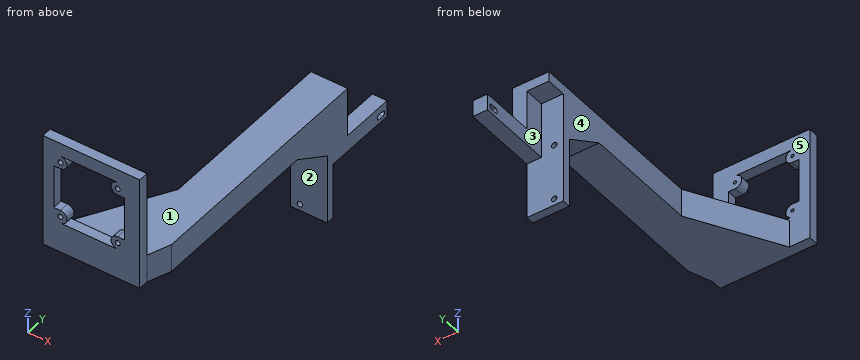
Autodesk Inventor part; units mm, degrees
ref_plane "YZ Plane" through (0, 0, 0) normal (1, 0, 0) x (0, 1, 0)
ref_plane "XZ Plane" through (0, 0, 0) normal (0, 1, 0) x (-1, 0, 0)
ref_plane "XY Plane" through (0, 0, 0) normal (0, 0, 1) x (1, 0, 0)
sketch "Sketch1" plane through (0, 0, 0) normal (0, 1, 0) x (-1, 0, 0)
  line L0 (0, 0) -> (13, 0)
  line L1 (13, 0) -> (13, -44)
  line L2 (13, -44) -> (0, -44)
  line L3 (0, -44) -> (0, 0)
  line L4 (13, 0) -> (13, -6)
  line L5 (13, -6) -> (7.5, -6)
  line L6 (7.5, -6) -> (7.5, -40)
  circle A0 centre (7.5, -6) radius 1.65
  circle A1 centre (7.5, -40) radius 1.65
  dimension "d0" = 13
  dimension "d1" = 44
  dimension "d2" = 6
  dimension "d3" = 5.5
  dimension "d4" = 34
  dimension "d5" = 3.3
  dimension "d6" = 3.3
extrude "Extrusion1" add sketch "Sketch1" along normal blind 5
sketch "Sketch2" plane through (0, 0, 0) normal (1, 0, 0) x (0, 0, -1)
  line L0 (0, 5) -> (44, 5)
  line L1 (0, 5) -> (44, 5)
  line L2 (44, 5) -> (44, 50)
  line L3 (44, 50) -> (0, 50)
  line L4 (0, 50) -> (0, 5)
  line L5 (0, 0) -> (44, 0)
  line L6 (44, 0) -> (44, 5)
  line L7 (44, 5) -> (0, 5)
  line L8 (0, 5) -> (0, 0)
  line L9 (0, 50) -> (10, 50)
  line L10 (10, 50) -> (10, 5)
  line L11 (10, 5) -> (0, 5)
  line L12 (0, 5) -> (0, 50)
  dimension "d9" = 44
  dimension "d10" = 45
  dimension "d11" = 10
extrude "Extrusion2" add sketch "Sketch2" along normal blind 4 contours L4 L3 L10 L0 | L0 L6 L5 L8
sketch "Sketch3" plane through (4, 0, 0) normal (1, 0, 0) x (0, 0, -1)
  line L0 (44, 5) -> (10, 5)
  line L1 (10, 5) -> (10, 45)
  line L2 (10, 5) -> (10, 50)
  line L3 (0, 50) -> (0, 5)
  line L4 (0, 45) -> (4.4, 45)
  line L5 (6, 45) -> (6, 46.5)
  line L6 (6, 45) -> (6, 43.5)
  line L7 (4.4, 46.5) -> (4.4, 43.5)
  line L8 (7.6, 46.5) -> (7.6, 43.5)
  arc A0 (5.4432, 45) -> (6, 44.9) centre (6, 46.5) ccw
  arc A1 (6.5568, 45) -> (4.4, 46.5) centre (6, 46.5) ccw
  line L9 (10, 45) -> (6.5568, 45)
  line L10 (5.4432, 45) -> (0, 45)
  arc A2 (6, 45.1) -> (5.4432, 45) centre (6, 43.5) ccw
  arc A3 (4.4, 43.5) -> (7.6, 43.5) centre (6, 43.5) ccw
  point P0 (0, 0)
  dimension "d14" = 40
  dimension "d15" = 6
  dimension "d16" = 1.5
  dimension "d17" = 1.5
extrude "Extrusion3" cut sketch "Sketch3" against normal blind 4 contours L6 A0 A2 L5 | A1 L9 L8 A3 L7 | L8 L9 A1
sketch "Sketch4" plane through (-13, 0, 0) normal (0, 0, 1) x (1, 0, 0)
  line L0 (0, 0) -> (17, 0)
  line L1 (17, 0) -> (17, 5)
  line L2 (0, 0) -> (17, 0)
  line L3 (17, 0) -> (17, 5)
  line L4 (17, 5) -> (0, 5)
  line L5 (0, 5) -> (0, 0)
  line L6 (13, 50) -> (13, 5)
  line L7 (17, 0) -> (13, 0)
  line L8 (13, 0) -> (13, 17)
  line L9 (13, 17) -> (17, 17)
  line L10 (17, 17) -> (17, 0)
  dimension "d22" = 17
extrude "Extrusion4" add sketch "Sketch4" along normal blind 30
sketch "Sketch5" plane through (0, 0, 0) normal (0, -1, 0) x (1, 0, 0)
  line L0 (-13, -44) -> (-13, 30)
  line L1 (-13, 30) -> (4, 30)
  line L2 (4, 30) -> (4, 13)
  line L3 (4, 13) -> (-13, 13)
  line L4 (-13, 13) -> (-13, 30)
  point P0 (0, 0)
  dimension "d25" = 17
  dimension "d26" = 17
extrude "Extrusion5" add sketch "Sketch5" along normal blind 150
sketch "Sketch7" plane through (0, -150, 0) normal (0, -1, 0) x (1, 0, 0)
  line L0 (4, 13) -> (-13, 13)
  line L1 (0, 30) -> (0, -10)
  line L2 (0, 13) -> (0, 30)
  line L3 (0, 30) -> (0, 52.6)
  circle A0 centre (-36, 52.6) radius 9
  line L4 (-36, 52.6) -> (-36, 36.6)
  line L5 (-36, 36.6) -> (-20, 36.6)
  line L6 (-36, 52.6) -> (-36, 68.6)
  line L7 (-36, 68.6) -> (-52, 68.6)
  line L8 (-52, 68.6) -> (-20, 68.6)
  line L9 (-20, 68.6) -> (-20, 36.6)
  line L10 (-20, 36.6) -> (-52, 36.6)
  line L11 (-52, 36.6) -> (-52, 68.6)
  circle A1 centre (-20, 68.6) radius 1.1
  circle A2 centre (-20, 36.6) radius 1.1
  circle A3 centre (-52, 36.6) radius 1.1
  circle A4 centre (-52, 68.6) radius 1.1
  circle A5 centre (-20, 68.6) radius 4
  circle A6 centre (-20, 36.6) radius 4
  line L12 (-52, 65.6) -> (-52, 70.6)
  line L13 (-52, 36.6) -> (-52, 42.6)
  circle A7 centre (-52, 68.6) radius 4
  circle A8 centre (-52, 36.6) radius 4
  point P0 (0, 0)
  point P1 (-20, 64.6)
  point P2 (-20, 40.6)
  dimension "d29" = 22.6
  dimension "d31" = 18
  dimension "d32" = 16
  dimension "d33" = 16
  dimension "d34" = 16
  dimension "d35" = 16
  dimension "d36" = 2.2
  dimension "d37" = 2.2
  dimension "d39" = 2.2
  dimension "d40" = 8
  dimension "d43" = 8
  dimension "d49" = 8
  dimension "d50" = 8
sketch "Sketch14" plane through (0, -150, 0) normal (0, -1, 0) x (1, 0, 0)
  line L0 (4, 13) -> (4, 30)
  line L1 (4, 13) -> (4, 52.6)
  line L2 (4, 52.6) -> (-26.5, 52.6)
  line L3 (-26.5, 52.6) -> (-26.5, 35.35)
  line L4 (-26.5, 35.35) -> (-9.25, 35.35)
  line L5 (-26.5, 52.6) -> (-43.75, 52.6)
  line L6 (-43.75, 52.6) -> (-43.75, 69.85)
  line L7 (-43.75, 69.85) -> (-9.25, 69.85)
  line L8 (-9.25, 69.85) -> (-9.25, 35.35)
  line L9 (-9.25, 35.35) -> (-43.75, 35.35)
  line L10 (-43.75, 35.35) -> (-43.75, 69.85)
  circle A0 centre (-43.75, 69.85) radius 0.95
  circle A1 centre (-9.25, 69.85) radius 0.95
  circle A2 centre (-9.25, 35.35) radius 0.95
  circle A3 centre (-43.75, 35.35) radius 0.95
  circle A4 centre (-43.75, 69.85) radius 4
  circle A5 centre (-9.25, 69.85) radius 4
  circle A6 centre (-9.25, 35.35) radius 4
  circle A7 centre (-43.75, 35.35) radius 4
  point P0 (0, 0)
  dimension "d91" = 39.6
  dimension "d92" = 30.5
  dimension "d93" = 17.25
  dimension "d94" = 17.25
  dimension "d95" = 17.25
  dimension "d96" = 17.25
  dimension "d97" = 1.9
  dimension "d98" = 1.9
  dimension "d99" = 1.9
  dimension "d100" = 1.9
  dimension "d101" = 8
  dimension "d102" = 8
  dimension "d103" = 8
  dimension "d104" = 8
extrude "Extrusion14" add sketch "Sketch14" against normal blind 6 contours A5 L7 A1 L8 | L8 A1 L7 A5 | A6 L4 A2 L8 | L8 A2 L4 A6 | A7 L10 A3 L9 | L9 A3 L10 A7 | A4 L7 A0 L6 | L6 A0 L7 A4
sketch "Sketch15" plane through (-9.25, -150, 69.85) normal (0, -1, 0) x (1, 0, 0)
  circle A0 centre (0, 0) radius 4
  line L0 (0, 4) -> (10, 4)
  line L1 (10, 4) -> (10, -4)
  line L2 (10, -4) -> (0, -4)
  line L3 (0, -4) -> (0, 4)
  circle A1 centre (0, -34.5) radius 4
  line L4 (0, -30.5) -> (10, -30.5)
  line L5 (10, -30.5) -> (10, -38.5)
  line L6 (10, -38.5) -> (0, -38.5)
  line L7 (0, -38.5) -> (0, -30.5)
  circle A2 centre (-34.5, -34.5) radius 4
  line L8 (-34.5, -38.5) -> (-44.5, -38.5)
  line L9 (-44.5, -38.5) -> (-44.5, -30.5)
  line L10 (-44.5, -30.5) -> (-34.5, -30.5)
  line L11 (-34.5, -30.5) -> (-34.5, -38.5)
  circle A3 centre (-34.5, 0) radius 4
  line L12 (-34.5, -4) -> (-44.5, -4)
  line L13 (-44.5, -4) -> (-44.5, 4)
  line L14 (-44.5, 4) -> (-34.5, 4)
  line L15 (-34.5, 4) -> (-34.5, -4)
  line L16 (-44.5, 4) -> (-38.5, 4)
  line L17 (-38.5, 4) -> (-38.5, -38.5)
  line L18 (-38.5, -38.5) -> (-44.5, -38.5)
  line L19 (-44.5, -38.5) -> (-44.5, 4)
  line L20 (10, 4) -> (4, 4)
  line L21 (4, 4) -> (4, -38.5)
  line L22 (4, -38.5) -> (10, -38.5)
  line L23 (10, -38.5) -> (10, 4)
  point P0 (9.25, -69.85)
  point P1 (-38.5, -4)
  point P2 (-34.5, 4)
  point P3 (-34.5, -30.5)
  point P4 (-38.5, -30.5)
  point P5 (0, -4)
  point P6 (4, -4)
  point P7 (4, -30.5)
  point P8 (0, -38.5)
  point P9 (10, -4)
  dimension "d107" = 10
  dimension "d108" = 8
  dimension "d109" = 10
  dimension "d110" = 8
  dimension "d111" = 10
  dimension "d112" = 8
  dimension "d113" = 10
  dimension "d114" = 8
  dimension "d115" = 6
  dimension "d116" = 6
extrude "Extrusion15" add sketch "Sketch15" against normal blind 6 contours L21 L2 A0 | A0 L0 L21 | L21 L0 L1 L2 | L2 L23 L4 L21 | L21 A1 L4 | L4 L5 L6 L21 | L21 L6 A1 | A2 L17 L10 | L8 L17 A2 | L17 L8 L9 L10 | L10 L19 L12 L17 | L17 A3 L12 | L12 L13 L14 L17 | L17 L14 A3
sketch "Sketch16" plane through (0, -150, 0) normal (0, -1, 0) x (1, 0, 0)
  line L0 (0.75, 73.85) -> (0.75, 31.35)
  line L1 (0.75, 73.85) -> (-51.25, 73.85)
  line L2 (-51.25, 73.85) -> (-51.25, 81.85)
  line L3 (-51.25, 81.85) -> (0.75, 81.85)
  line L4 (0.75, 81.85) -> (0.75, 73.85)
  line L5 (0.75, 31.35) -> (-9.25, 31.35)
  line L6 (0.75, 31.35) -> (-51.25, 31.35)
  line L7 (-51.25, 31.35) -> (-51.25, 23.35)
  line L8 (-51.25, 23.35) -> (0.75, 23.35)
  line L9 (0.75, 23.35) -> (0.75, 31.35)
  point P0 (0, 0)
  dimension "d119" = 8
  dimension "d120" = 8
extrude "Extrusion16" add sketch "Sketch16" against normal blind 6
sketch "Sketch17" plane through (0, -144, 0) normal (0, 1, 0) x (1, 0, 0)
  line L0 (0.75, -81.85) -> (0.75, -30)
  line L1 (4, -30) -> (0, -30)
  line L2 (0.75, -81.85) -> (4, -81.85)
  line L3 (4, -81.85) -> (4, -30)
  line L4 (4, -30) -> (0.75, -30)
  line L5 (0.75, -30) -> (0.75, -81.85)
  line L6 (-51.25, -23.35) -> (-51.25, -81.85)
  line L7 (-51.25, -23.35) -> (-13, -23.35)
  line L8 (-13, -23.35) -> (-13, -13)
  line L9 (-13, -13) -> (-51.25, -13)
  line L10 (-51.25, -13) -> (-51.25, -23.35)
  point P0 (0, 0)
  point P1 (0.75, -30)
  point P2 (0.75, -30)
extrude "Extrusion17" add sketch "Sketch17" against normal blind 6
chamfer "Chamfer4" distance 50 angle 30 1 edges at (-13, -144, 21.5) measured on face at (-13, -46.3333, 24.3333)
chamfer "Chamfer5" distance 25 angle 30 1 edges at (-4.5, 0, 13) measured on face at (-1.6667, -81.3333, 13)
sketch "Sketch19" plane through (-13, 0, 30) normal (0, 0, 1) x (1, 0, 0)
  line L0 (13, 17) -> (13, 5)
  line L1 (0, 0) -> (0, 5)
  line L2 (13, 17) -> (0, 17)
  line L3 (0, 17) -> (0, 5)
  line L4 (0, 5) -> (13, 5)
  line L5 (13, 5) -> (13, 17)
  point P0 (13, 0)
extrude "Extrusion18" add sketch "Sketch19" against normal blind 6
sketch "Sketch20" plane through (-51.25, -150, 13) normal (-1, 0, 0) x (0, 0, 1)
  line L0 (0, 125) -> (0, 0)
  line L1 (60.85, 6) -> (68.85, 6)
  line L2 (0, 0) -> (68.85, 0)
  line L3 (68.85, 0) -> (68.85, 6)
  line L4 (68.85, 6) -> (0, 6)
  line L5 (0, 6) -> (0, 0)
  point P0 (-13, 150)
extrude "Extrusion19" add sketch "Sketch20" along normal blind 3
sketch "Sketch21" plane through (0, 0, 0) normal (-1, 0, 0) x (0, 0, 1)
  line L0 (-10, 5) -> (-10, 50)
  line L1 (24, 5) -> (-10, 5)
  line L2 (-10, 50) -> (24, 50)
  line L3 (24, 50) -> (24, 5)
  line L4 (24, 5) -> (-10, 5)
  line L5 (-10, 5) -> (-10, 50)
  point P0 (0, 0)
extrude "Extrusion20" cut sketch "Sketch21" against normal blind 0.2
chamfer "Chamfer6" distance 2 angle 15 1 edges at (-10.2, -150, 69.85) measured on face at (-8.3489, -146, 69.5492)
chamfer "Chamfer7" distance 2 angle 15 1 edges at (-10.2, -150, 35.35) measured on face at (-8.6492, -146, 36.0859)
chamfer "Chamfer8" distance 2 angle 15 1 edges at (-44.7, -150, 35.35) measured on face at (-43.7117, -146, 34.4008)
chamfer "Chamfer9" distance 2 angle 15 1 edges at (-44.7, -150, 69.85) measured on face at (-42.8489, -146, 69.5492)
sketch "Sketch22" plane through (4, 0, 0) normal (1, 0, 0) x (0, 0, -1)
  line L0 (44, 0) -> (1.4338, 0)
  line L1 (-30, 17) -> (-30, -144)
  line L2 (44, 0) -> (-30, 0)
  line L3 (-30, 0) -> (-30, 17)
  line L4 (-30, 17) -> (44, 17)
  line L5 (44, 17) -> (44, 0)
  line L6 (10, 50) -> (0, 50)
  line L7 (10, 50) -> (0, 50)
  line L8 (0, 50) -> (0, 0)
  line L9 (0, 0) -> (10, 0)
  line L10 (10, 0) -> (10, 50)
  line L11 (10, 5) -> (10, 50)
  line L12 (44, 17) -> (10, 17)
  line L13 (10, 17) -> (10, 5)
  line L14 (10, 5) -> (44, 5)
  line L15 (44, 5) -> (44, 17)
  arc A0 (4.4, 43.5) -> (7.6, 43.5) centre (6, 43.5) ccw
  circle A1 centre (6, 43.5) radius 1.6
  arc A2 (7.6, 46.5) -> (4.4, 46.5) centre (6, 46.5) ccw
  circle A3 centre (6, 46.5) radius 1.6
  line L16 (7.6, 46.5) -> (7.6, 43.5)
  line L17 (7.6, 46.5) -> (7.6, 43.5)
  line L18 (7.6, 43.5) -> (4.4, 43.5)
  line L19 (4.4, 43.5) -> (4.4, 46.5)
  line L20 (4.4, 46.5) -> (4.4, 43.5)
  point P0 (0, 17)
  point P1 (1.4338, 0)
extrude "Extrusion21" add sketch "Sketch22" along normal blind 5 contours L0 L10 L14 L5 | L0 L2 L8 L4 L10 | L2 L1 L4 L8 | L4 L8 L6 L10
sketch "Sketch23" plane through (4, 0, 0) normal (1, 0, 0) x (0, 0, -1)
  line L0 (-13, -25) -> (-13, -94)
  line L1 (-13, -25) -> (1.4338, 0)
  line L2 (-13, -25) -> (1.4338, 0)
  line L3 (-30, 0) -> (44, 0)
  line L4 (1.4338, 0) -> (-30, 0)
  line L5 (-30, 0) -> (-30, -144)
  line L6 (-30, 0) -> (-30, -144)
  line L7 (-81.85, -144) -> (-13, -144)
  line L8 (-30, -144) -> (-13, -144)
  line L9 (-13, -144) -> (-13, -25)
  point P0 (0, 0)
extrude "Extrusion22" add sketch "Sketch23" along normal blind 5
chamfer "Chamfer10" distance 13.737 angle 20 1 edges at (9, -144, 21.5) measured on face at (9, -50.6667, 24.3333)
properties part number "camera_mount_v2"
Geometry check sheet. Reference: the model listing, model coordinates, mm. Face numbers are marked on the shaded views. A direction names the side the tool comes from. Give positions to 0.01 mm unless a question says otherwise; leave off trailing zeros. Write each loop counter-clockwise with the first axis right and the second up, starting at its lowest first coordinate (ties: lowest second). Pieces come first, ordered by that corner, then holes.
1) Section check A-A, the plane x = -3. Record the boundary of the cut face in (y, z).
2) Section check B-B, the plane z = -33.5. Record the boundary of the cut face in (x, y).
3) Section check D-D, the plane y = -91. Record the boundary of the cut face in (x, z).
4) Section check C-C, the plane y = -20.5. Record the boundary of the cut face in (x, z), and give its area (3 significant figures).
5) Gauge pin test, flat ends, axial feed: pin 1 (1.5 mm diameter, centred on x = 4.5, y = 45.5, fed in from -Z); pin 2 (22 mm diameter, centred on y = -30, z = 1.5, fed in from -X); pin 3 (11 mm diameter, centred on x = -3, z = 19, fed in from +Y); pin 4 (0.9 mm diameter, centred on x = 4, y = 45, fed in from +Z). Record the tip position at first contact, or that the pin passes through.
6) Material ranges on L1, parallel to X at y = -145.6, z = 69.85; L2, parallel to Z at x = -7.5, y = 3.7; L3, parallel to Z at x = -9, y = -145, recorded low to high.
7) Access from +Z, -Z, +X, -X, +Y, -Y to the whole of each face (thin tool, end or side, straight path). Record for the marked faces 1, 2, 3, 4 and 5.
Computed:
1. outline: (-150, 13) - (-25, 13) - (0, -1.43) - (0, -44) - (5, -44) - (5, 24) - (17, 24) - (17, 30) - (-144, 30) - (-144, 81.85) - (-150, 81.85) - close
2. outline: (-13, 0) - (9, 0) - (9, 5) - (-13, 5) - close
3. outline: (-13, 13) - (9, 13) - (9, 30) - (-13, 30) - close
4. outline: (-13, 10.4) - (9, 10.4) - (9, 30) - (-13, 30) - close
4. area: 431 mm2
5. pin 1: stops at z = -10
5. pin 2: passes through
5. pin 3: stops at y = 17
5. pin 4: stops at z = 0
6. L1: x = -54.25 to -44.7, -42.8 to -39.75, -13.25 to -10.2, -8.3 to 4
6. L2: z = -44 to -41.65, -38.35 to -7.65, -4.35 to 30
6. L3: z = 13 to 34.43, 36.27 to 39.35, 65.85 to 68.93, 70.77 to 81.85
7. face 1: +Z, +X, -X, +Y
7. face 2: -Z, +X, -X, -Y
7. face 3: -Z, -X, +Y
7. face 4: +Z, -Z, -X, +Y
7. face 5: +Z, -X, +Y
